```python
from build123d import *

# Parameters (mm, degrees)
ESBO_O1_R                = 1.5
RESSALTO_EXTRUS_O1_DEPTH = 3


with BuildPart() as part:
    # Esboço1 → Ressalto-extrusão1 (new body)
    with BuildSketch(Plane.XY):
        with BuildLine():
            Line((3.125, -119.95), (3.125, -125.1))
            Line((3.125, -125.1), (9.5, -125.1))
            Line((9.5, -125.1), (9.051444859, -118.948386637))
            ThreePointArc((9.051444859, -118.948386637), (8.249352939, -77.177382145), (11.920153881, -35.560253603))
            Line((11.920153881, -35.560253603), (12, -35))
            Line((12, -35), (12, -12.5))
            ThreePointArc((12, -12.5), (9.071067812, -5.428932188), (2, -2.5))
            Line((2, -2.5), (0, -2.5))
            Line((0, -2.5), (-2, -2.5))
            ThreePointArc((-2, -2.5), (-9.071067812, -5.428932188), (-12, -12.5))
            Line((-12, -12.5), (-12, -35))
            Line((-12, -35), (-11.920153926, -35.560253285))
            ThreePointArc((-11.920153926, -35.560253285), (-8.249352944, -77.177381984), (-9.051444859, -118.948386634))
            Line((-9.051444859, -118.948386634), (-9.5, -125.1))
            Line((-9.5, -125.1), (-3.125, -125.1))
            Line((-3.125, -125.1), (-3.125, -119.95))
            Line((-3.125, -119.95), (-1.5, -119.95))
            Line((-1.5, -119.95), (-1.5, -115.1))
            Line((-1.5, -115.1), (1.5, -115.1))
            Line((1.5, -115.1), (1.5, -119.95))
            Line((1.5, -119.95), (3.125, -119.95))
        make_face()
        with Locations(Location((0, -8.5, 0), (0, 0, 180))):
            Circle(ESBO_O1_R, mode=Mode.SUBTRACT)
        with Locations(Location((0, -38.499871023, 0), (0, 0, 180))):
            Circle(ESBO_O1_R, mode=Mode.SUBTRACT)
        Polygon((-6, -23.5), (-6, -12), (6, -12), (6, -35), (2.474745195, -35), (-2.5, -35), (-6, -35), align=None, mode=Mode.SUBTRACT)
    extrude(amount=RESSALTO_EXTRUS_O1_DEPTH)


solid = part.part
```
For this review, take the finished solid that the model builds, in its own axes (mm). A direction names the side the tool comes from. Round coordinates to 2 decimals unless told otherwise and drop trailing zeros. Write each loop counter-clockwise with the first axis right and the second up, starting at its lowest first coordinate (ties: lowest second). Pieces come first, ordered by that corner, then holes. Notation, with made-up numbers: (70.5, -18.75) - (129.5, -18.75) arc R29 ccw to (129.5, 5.25) - close; hole circle Ø7 at (39.5, -25). An arc over 180 degrees is marked (long way). Answer as CSV lines item,"result". Start each with the question number.
(1) Add section B-B, the plane x = 0. State the section outline as (y, z) points, plus the area to 3 significant figures.
(2) Machinability: for faces 1 (the flat face through (6, -23, 1)), 2 (the flat face through (-9.273, -121.981, 1.479)), 3 (the flat face through (-1.5, -118, 1)), 4 (the flat face through (9.28, -122.07, 1.48)), which of the approach directions +Z, -Z, +X, -X, +Y, -Y give a long, thin tool a straight path to every point of the face, cutting with its end or side? Answer none if there is none.
(3) For pin 1 (1.5 mm diameter, centred on y = -118, z = 1.5, fed in from +X); pin 2 (1.5 mm diameter, centred on y = -121.5, z = 2, fed in from +X); pin 3 (1 mm diameter, centred on y = -81.5, z = 0.5, fed in from +X), all flat-tipped, find the tip position at first contact; note any pin that passes through.
(4) Add section A-A, the plane y = -22.5. State the section outline as (x, z) points.
(5) Add section D-D, the plane y = -8.5. State the section outline as (x, z) points, plus the area to 3 significant figures.
(6) Add section C-C, the plane z = 1.7. State the section outline as (x, y) points (3 decimals), plus the area to 3 significant figures.
(7) For line 1 (Y direction, x = 0, z = 0.75); line 2 (X direction, y = -27, z = 1.45); line 3 (Y direction, x = 4, z = 1.5), list the stretches that pass through material, from the lowest coordinate up.
(8) Mouldability with a two-part tool opening along Y and no side actions: class faces 5 (the cylindrical face through (-8.99, -5.35, 1.48)), 6 (the flat face through (0, -115.1, 1)), 7 (the flat face through (12, -24, 1)), 8 (the cylindrical face through (0, -7, 1)) as +Y half, -Y half, draft (parallel to the pull), parting line (faces both ways), or undercut.
From the geometry:
1,outline,"(-115.1, 0) - (-40, 0) - (-40, 3) - (-115.1, 3) - close; (-37, 0) - (-35, 0) - (-35, 3) - (-37, 3) - close; (-12, 0) - (-10, 0) - (-10, 3) - (-12, 3) - close; (-7, 0) - (-2.5, 0) - (-2.5, 3) - (-7, 3) - close"
1,area,"251 mm²"
2,face 1,"+Z, -Z"
2,face 2,"+Z, -Z, -X"
2,face 3,"+Z, -Z, -Y"
2,face 4,"+Z, -Z, +X"
3,pin 1,"stops at x = 9.04"
3,pin 2,"stops at x = 9.29"
3,pin 3,"stops at x = 8.14"
4,outline,"(-12, 0) - (-6, 0) - (-6, 3) - (-12, 3) - close; (6, 0) - (12, 0) - (12, 3) - (6, 3) - close"
5,outline,"(-11.17, 0) - (-1.5, 0) - (-1.5, 3) - (-11.17, 3) - close; (1.5, 0) - (11.17, 0) - (11.17, 3) - (1.5, 3) - close"
5,area,"58.0 mm²"
6,outline,"(-12, -35) - (-11.92, -35.56) arc R390 cw to (-9.051, -118.948) - (-9.5, -125.1) - (-3.125, -125.1) - (-3.125, -119.95) - (-1.5, -119.95) - (-1.5, -115.1) - (1.5, -115.1) - (1.5, -119.95) - (3.125, -119.95) - (3.125, -125.1) - (9.5, -125.1) - (9.051, -118.948) arc R390 cw to (11.92, -35.56) - (12, -35) - (12, -12.5) arc R10 ccw to (2, -2.5) - (-2, -2.5) arc R10 ccw to (-12, -12.5) - close; hole (-6, -35) - (6, -35) - (6, -12) - (-6, -12) - close; hole circle Ø3 at (0, -38.5); hole circle Ø3 at (0, -8.5)"
6,area,"2,030 mm²"
7,line 1,"y = -115.1 to -40, -37 to -35, -12 to -10, -7 to -2.5"
7,line 2,"x = -12 to -6, 6 to 12"
7,line 3,"y = -125.1 to -35, -12 to -2.7"
8,face 5,"+Y half"
8,face 6,"-Y half"
8,face 7,"draft"
8,face 8,"undercut"
